from build123d import *

# Parameters (mm, degrees)
F4_R          = 2.9337
F5_DEPTH      = 14.0716
F4_W          = 19.6088
F4_H          = 39.9542
F6_DEPTH      = 8.255
F6_DEPTH_BACK = 30.9626
F4_H_2        = 7.3152
F4_R_2        = 2.1336
F7_DEPTH      = 3.4798
F9_W          = 6.6548
F9_H          = 4.318
F10_DEPTH     = 7.62


# Not quite as in the source:
# - a variable given as a bare number and used for a length is read in inches; the dataset says mm whatever the document's units were


with BuildPart() as f5:
    # F4 (on Top) → F5 (new body)
    with BuildSketch(Plane.XY):
        with Locations((0, 10.1727)):
            Circle(F4_R)
    extrude(amount=F5_DEPTH)

    # F4 (on Top) → F6 (join, two sides)
    with BuildSketch(Plane.XY) as f6_sk:
        Rectangle(F4_W, F4_H)
        with Locations((0, 10.1727)):
            Circle(F4_R, mode=Mode.SUBTRACT)
        with Locations((0, 10.1727)):
            Circle(F4_R)
    extrude(amount=F6_DEPTH)
    extrude(f6_sk.sketch, amount=-F6_DEPTH_BACK)

    # F4 (on Top) → F7 (join)
    with BuildSketch(Plane.XY):
        with Locations((0, 23.6347)):
            Rectangle(F4_W, F4_H_2)
        with Locations((-5.1308, 24.3967)):
            Circle(F4_R_2, mode=Mode.SUBTRACT)
        with Locations((5.1308, 24.3967)):
            Circle(F4_R_2, mode=Mode.SUBTRACT)
        with Locations((0, -23.6347)):
            Rectangle(F4_W, F4_H_2)
        with Locations((-5.1308, -24.3967)):
            Circle(F4_R_2, mode=Mode.SUBTRACT)
        with Locations((5.1308, -24.3967)):
            Circle(F4_R_2, mode=Mode.SUBTRACT)
    extrude(amount=-F7_DEPTH)

    # F9 (on face) → F10 (join)
    with BuildSketch(Plane(origin=(0, 19.9771, 0), x_dir=(-1, 0, 0), z_dir=(0, 1, 0))):
        with Locations((0, -25.5016)):
            Rectangle(F9_W, F9_H)
    extrude(amount=F10_DEPTH)


solid = f5.part
Work out the finished part from the listing and answer in its coordinate system (mm). A direction names the side the tool comes from. Coordinates: 2 decimals unless noted, no trailing zeros. Write each loop counter-clockwise with the first axis right and the second up, starting at its lowest first coordinate (ties: lowest second). Pieces come first, ordered by that corner, then holes. Notation, with made-up numbers: (38, -30) - (47, -30) arc R26 ccw to (47, -16) - close; hole circle Ø1 at (57.5, -39). An arc over 180 degrees is marked (long way). One line per question, with ' | ' between items.
1) Consider probe 1 along Y at (x, z) = (-6, -14); probe 2 along Z at (x, y) = (1.5, 18.5) (3 decimals); probe 3 along Y at (x, z) = (-1, -1). Determine where each line is inside the solid, lowest interval first. Write a range as [from, to].
Checks:
probe 1: [-19.98, 19.98] | probe 2: [-30.963, 8.255] | probe 3: [-27.29, 27.29]
2) For faces 4 (the face through (0, 24, -23.343)), 5 (the face through (3.327, 24, -26)), 6 (the face through (0, 24, 0)), 7 (the face through (-3.327, 24, -26)), 8 (the face through (0, -24, -3.48)), determine the directions among +Z, -Z, +X, -X, +Y, -Y from which every point of the face is accessible in a straight line to the end or side of a thin tool.
Checks:
face 4: +X, -X, +Y | face 5: -Z, +X, +Y | face 6: +Z, +X, -X, +Y | face 7: -Z, -X, +Y | face 8: -Z, +X, -X, -Y
3) Find section B-B, the plane z = -25. Determine the outline of the cut face in (x, y).
Checks:
outline: (-9.8, -19.98) - (9.8, -19.98) - (9.8, 19.98) - (3.33, 19.98) - (3.33, 27.6) - (-3.33, 27.6) - (-3.33, 19.98) - (-9.8, 19.98) - close
4) Flat-ended cylindrical pins translate along their axes: P1, Ø2.5, axis at x = 5.13, y = -24.4, coming from the -Z side; P2, Ø5.5, axis at x = 0, y = 25, coming from the +Z side; P3, Ø1.3, axis at y = 25, z = -25, coming from the +X side; P4, Ø1, axis at x = -3, z = -10.5, coming from the -Y side. Find the tip coordinate at first contact, or state that the pin passes through.
Checks:
P1: through | P2: z = 0 | P3: x = 3.33 | P4: y = -19.98
5) Find section A-A, the plane x = 0. Determine the outline of the cut face in (y, z) (3 decimals).
Checks:
outline: (-27.292, -3.48) - (-19.977, -3.48) - (-19.977, -30.963) - (19.977, -30.963) - (19.977, -27.661) - (27.597, -27.661) - (27.597, -23.343) - (19.977, -23.343) - (19.977, -3.48) - (27.292, -3.48) - (27.292, 0) - (19.977, 0) - (19.977, 8.255) - (13.106, 8.255) - (13.106, 14.072) - (7.239, 14.072) - (7.239, 8.255) - (-19.977, 8.255) - (-19.977, 0) - (-27.292, 0) - close
6) Find section C-C, the plane x = -4.5. Determine the outline of the cut face in (y, z) (3 decimals), and give its area (3 significant figures).
Checks:
outline: (-27.292, -3.48) - (-26.435, -3.48) - (-26.435, 0) - (-27.292, 0) - close; (-22.358, -3.48) - (-19.977, -3.48) - (-19.977, -30.963) - (19.977, -30.963) - (19.977, -3.48) - (22.358, -3.48) - (22.358, 0) - (19.977, 0) - (19.977, 8.255) - (-19.977, 8.255) - (-19.977, 0) - (-22.358, 0) - close; (26.435, -3.48) - (27.292, -3.48) - (27.292, 0) - (26.435, 0) - close | area: 1,590 mm2
7) Find section D-D, the plane y = -2.5. Determine the outline of the cut face in (x, z) (3 decimals).
Checks:
outline: (-9.804, -30.963) - (9.804, -30.963) - (9.804, 8.255) - (-9.804, 8.255) - close
8) The mould has two halves that part along Y. Classify faces 1 (the face through (0, 27.597, -25)), 2 (the face through (-5.41, -22.28, -1.72)), 3 (the face through (0, -24, 0)): +Y half, -Y half, draft (parallel to the pull), parting line (faces both ways), or undercut.
Checks:
face 1: +Y half | face 2: undercut | face 3: draft
